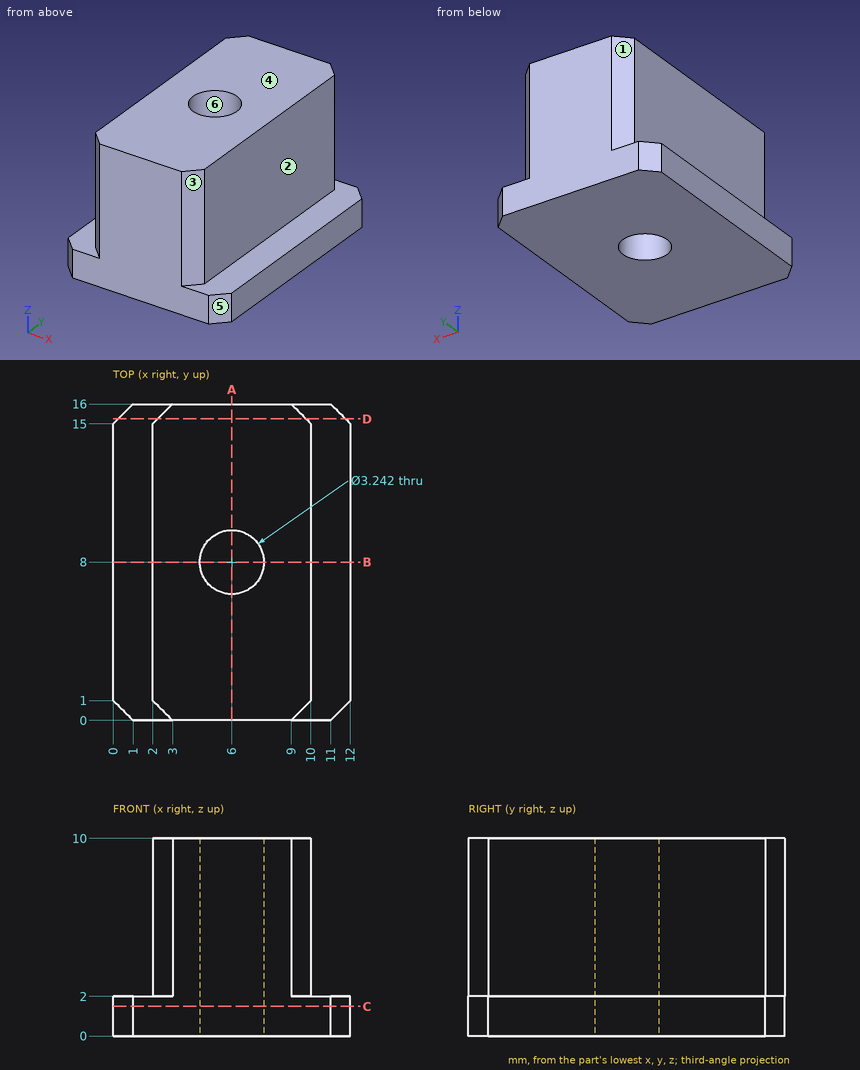
Check sheet for the drawn part. Datum: minimum x, y, z corner. Units: mm. A direction names the side the tool comes from. Round coordinates to 2 decimals unless told otherwise and drop trailing zeros. Write each loop counter-clockwise with the first axis right and the second up, starting at its lowest first coordinate (ties: lowest second). Pieces come first, ordered by that corner, then holes. Notation, with made-up numbers: (85, 58) -> (130, 58) arc R26 cw to (130, 85) -> close; hole circle Ø10 at (81.5, 59.5). An arc over 180 degrees is marked (long way). One line per item, written item: value. Start each with the question number.
(1) Cross-section at D-D, the plane y = 15.25. Record the cut outline in (x, z), and give its area (3 significant figures).
(2) Access from +Z, -Z, +X, -X, +Y, -Y to the whole of each face (thin tool, end or side, straight path). Record for the marked faces 1, 2 and 3.
(3) Draft check along X on the marked faces 4, 5 and 6. Enter one of: +X half, -X half, draft (parallel to the pull), parting line (faces both ways), or undercut.
(4) Cross-section at C-C, the plane z = 1.5. Record the cut outline in (x, y).
(5) Cross-section at A-A, the plane x = 6. Record the cut outline in (y, z).
(6) Scan lines: line 1 (Y direction, x = 6, z = 7.25); line 2 (X direction, y = 8, z = 7.75); line 3 (Z direction, x = 11.25, y = 9). Record each from-to range of solid material in increasing order. Write a range as [from, to].
(7) Cross-section at B-B, the plane y = 8. Record the cut outline in (x, z), and give its area (3 significant figures).
(8) Go/stop test with flat-tipped pins: pin 1 Ø1 at (x, y) = (6, 9) entering from -Z; pin 2 Ø1.5 at (y, z) = (5.5, 6) entering from -X; pin 3 Ø1.5 at (x, y) = (10.5, 9.5) entering from -Z; pin 4 Ø1 at (y, z) = (10, 7.5) entering from +X. Record where each tip stops, or that it passes through.
Answer:
1. outline: (0.25, 0) -> (11.75, 0) -> (11.75, 2) -> (9.75, 2) -> (9.75, 10) -> (2.25, 10) -> (2.25, 2) -> (0.25, 2) -> close
1. area: 83.0 mm²
2. face 1: +Z, -X, +Y
2. face 2: +Z, +X, +Y, -Y
2. face 3: +Z, +X, -Y
3. face 4: draft
3. face 5: +X half
3. face 6: undercut
4. outline: (0, 1) -> (1, 0) -> (11, 0) -> (12, 1) -> (12, 15) -> (11, 16) -> (1, 16) -> (0, 15) -> close; hole circle Ø3.24 at (6, 8)
5. outline: (0, 0) -> (6.38, 0) -> (6.38, 10) -> (0, 10) -> close; (9.62, 0) -> (16, 0) -> (16, 10) -> (9.62, 10) -> close
6. line 1: [0, 6.38], [9.62, 16]
6. line 2: [2, 4.38], [7.62, 10]
6. line 3: [0, 2]
7. outline: (0, 0) -> (4.38, 0) -> (4.38, 10) -> (2, 10) -> (2, 2) -> (0, 2) -> close; (7.62, 0) -> (12, 0) -> (12, 2) -> (10, 2) -> (10, 10) -> (7.62, 10) -> close
7. area: 55.6 mm²
8. pin 1: through
8. pin 2: x = 2
8. pin 3: z = 0
8. pin 4: x = 10
